Build history of the part. All positions in model axes, mm. A direction names the side the tool comes from. Round coordinates to 2 decimals unless told otherwise and drop trailing zeros. Write each loop counter-clockwise with the first axis right and the second up, starting at its lowest first coordinate (ties: lowest second). Pieces come first, ordered by that corner, then holes. Notation, with made-up numbers: (50, 26) - (77, 26) arc R10 ccw to (77, 43) - close; hole circle Ø10 at (60, -27). An arc over 180 degrees is marked (long way). One line per question, with ' | ' between items.
from build123d import *

# Parameters (mm, degrees)
BASE_FLANGIA1_DEPTH       = 272.5
BORDO_FLANGIA1_DEPTH      = 451
BORDO_FLANGIA1_BEND_DEPTH = 451


# Sheet-metal steps are written as plain solids
with BuildPart() as part:
    # Schizzo1 → Base-Flangia1 (new, symmetric)
    with BuildSketch(Plane.XY):
        with BuildLine():
            Line((-262.5, 50), (-235.5, 50))
            ThreePointArc((-235.5, 50), (-233.378679656, 49.121320344), (-232.5, 47))
            Line((-232.5, 47), (-232.5, 7))
            ThreePointArc((-232.5, 7), (-230.449747468, 2.050252532), (-225.5, 0))
            Line((-225.5, 0), (225.5, 0))
            ThreePointArc((225.5, 0), (230.449747468, 2.050252532), (232.5, 7))
            Line((232.5, 7), (232.5, 47))
            ThreePointArc((232.5, 47), (233.378679656, 49.121320344), (235.5, 50))
            Line((235.5, 50), (262.5, 50))
            Line((262.5, 50), (262.5, 54))
            Line((262.5, 54), (235.5, 54))
            ThreePointArc((235.5, 54), (230.550252532, 51.949747468), (228.5, 47))
            Line((228.5, 47), (228.5, 7))
            ThreePointArc((228.5, 7), (227.621320344, 4.878679656), (225.5, 4))
            Line((225.5, 4), (-225.5, 4))
            ThreePointArc((-225.5, 4), (-227.621320344, 4.878679656), (-228.5, 7))
            Line((-228.5, 7), (-228.5, 47))
            ThreePointArc((-228.5, 47), (-230.550252532, 51.949747468), (-235.5, 54))
            Line((-235.5, 54), (-262.5, 54))
            Line((-262.5, 54), (-262.5, 50))
        make_face()
    extrude(amount=BASE_FLANGIA1_DEPTH, both=True)

    # Bordo-Flangia1 section (across the edge) → Bordo-Flangia1 (add)
    with BuildSketch(Plane(origin=(-225.5, 4, 275.5), x_dir=(0, 0, -1), z_dir=(1, 0, 0))):
        with BuildLine():
            Line((-4, 3), (-4, 36))
            Line((-4, 36), (0, 36))
            Line((0, 36), (0, 3))
            ThreePointArc((0, 3), (0.878679656, 0.878679656), (3, 0))
            Line((3, 0), (3, -4))
            ThreePointArc((3, -4), (-1.949747468, -1.949747468), (-4, 3))
        make_face()
    extrude(amount=BORDO_FLANGIA1_DEPTH)

    # Bordo-Flangia1 section 2 (across the edge) → Bordo-Flangia1 bend (add)
    with BuildSketch(Plane(origin=(225.5, 4, -275.5), x_dir=(0, 0, 1), z_dir=(-1, 0, 0))):
        with BuildLine():
            Line((-4, 3), (-4, 36))
            Line((-4, 36), (0, 36))
            Line((0, 36), (0, 3))
            ThreePointArc((0, 3), (0.878679656, 0.878679656), (3, 0))
            Line((3, 0), (3, -4))
            ThreePointArc((3, -4), (-1.949747468, -1.949747468), (-4, 3))
        make_face()
    extrude(amount=BORDO_FLANGIA1_BEND_DEPTH)


solid = part.part
Q1. Saw through at A-A, the plane y = 24. List the corners of the cut face in (x, z).
Found:
outline: (-232.5, -272.5) - (-228.5, -272.5) - (-228.5, 272.5) - (-232.5, 272.5) - close; (-225.5, -279.5) - (225.5, -279.5) - (225.5, -275.5) - (-225.5, -275.5) - close; (-225.5, 275.5) - (225.5, 275.5) - (225.5, 279.5) - (-225.5, 279.5) - close; (228.5, -272.5) - (232.5, -272.5) - (232.5, 272.5) - (228.5, 272.5) - close
Q2. Drop flat-ended pins along their axis: pin 1 (3.5 mm diameter, centred on y = 17.5, z = -277.5, fed in from +X); pin 2 (1.2 mm diameter, centred on x = 90.5, z = 278.5, fed in from +Y); pin 3 (18.5 mm diameter, centred on x = -244.5, y = 14, fed in from -Z); pin 4 (18.5 mm diameter, centred on x = 235.5, y = 26, fed in from -Z). Give the stop position or say it passes through.
Found:
pin 1: x = 225.5 | pin 2: y = 40 | pin 3: through | pin 4: z = -272.5
Q3. Drill centre lines: L1, parallel to Z at x = 144, y = 39; L2, parallel to X at y = 31.5, z = -59; L3, parallel to Y at x = -178.5, z = -81.5. Where is each one in solid material? Low to high. Write a range as from..to.
Found:
L1: -279.5..-275.5, 275.5..279.5 | L2: -232.5..-228.5, 228.5..232.5 | L3: 0..4
Q4. Which spindle directions (+Z, -Z, +X, -X, +Y, -Y) get a long thin tool onto all of the face, cutting with end or side? Do faces 4 (the flat face through (-228.5, 27, 4)), 5 (the flat face through (3, 24, -275.5)), 6 (the flat face through (-249, 50, 4)). Say none if no direction does.
Found:
face 4: +Z, -Z, +Y | face 5: +X, -X, +Y | face 6: +Z, -Z, -X, -Y
Q5. Saw through at C-C, the plane x = 100.5. List the corners of the cut face in (y, z).
Found:
outline: (0, -272.5) arc R7 ccw to (7, -279.5) - (40, -279.5) - (40, -275.5) - (7, -275.5) arc R3 cw to (4, -272.5) - (4, 272.5) arc R3 cw to (7, 275.5) - (40, 275.5) - (40, 279.5) - (7, 279.5) arc R7 ccw to (0, 272.5) - close
Q6. Saw through at B-B, the plane z = 125.5. List the corners of the cut face in (x, y), then the cut area to 3 significant figures.
Found:
outline: (-262.5, 50) - (-235.5, 50) arc R3 cw to (-232.5, 47) - (-232.5, 7) arc R7 ccw to (-225.5, 0) - (225.5, 0) arc R7 ccw to (232.5, 7) - (232.5, 47) arc R3 cw to (235.5, 50) - (262.5, 50) - (262.5, 54) - (235.5, 54) arc R7 ccw to (228.5, 47) - (228.5, 7) arc R3 cw to (225.5, 4) - (-225.5, 4) arc R3 cw to (-228.5, 7) - (-228.5, 47) arc R7 ccw to (-235.5, 54) - (-262.5, 54) - close | area: 2,470 mm^2
Q7. Pull direction X, two halves, no side cores. Call faces 1 (the flat face through (228.5, 27, 4)), 2 (the flat face through (232.5, 27, 4)), 3 (the flat face through (-232, 35, 272.5)): +X half, -X half, draft (parallel to the pull), parting line (faces both ways), or undercut.
Found:
face 1: undercut | face 2: +X half | face 3: draft
